Could you check a few things on this drawing? It's one solid part, dimensions in mm from its lowest x, y, z. A direction names the side the tool comes from. Give positions to 0.01 mm unless a question says otherwise; leave off trailing zeros. Order: outer loops, then holes, each group sorted by start corner. A loop starts at its lowest first (then second) coordinate and runs counter-clockwise, first axis right, second up. Notation, with made-up numbers: M 22.5,-15.75 L 38.5,-15.75 A22 ccw 38.5,-5.75 Z; hole C 28.25,88 d6. An arc over 180 degrees is marked long. Use one line per item in the form item = value.
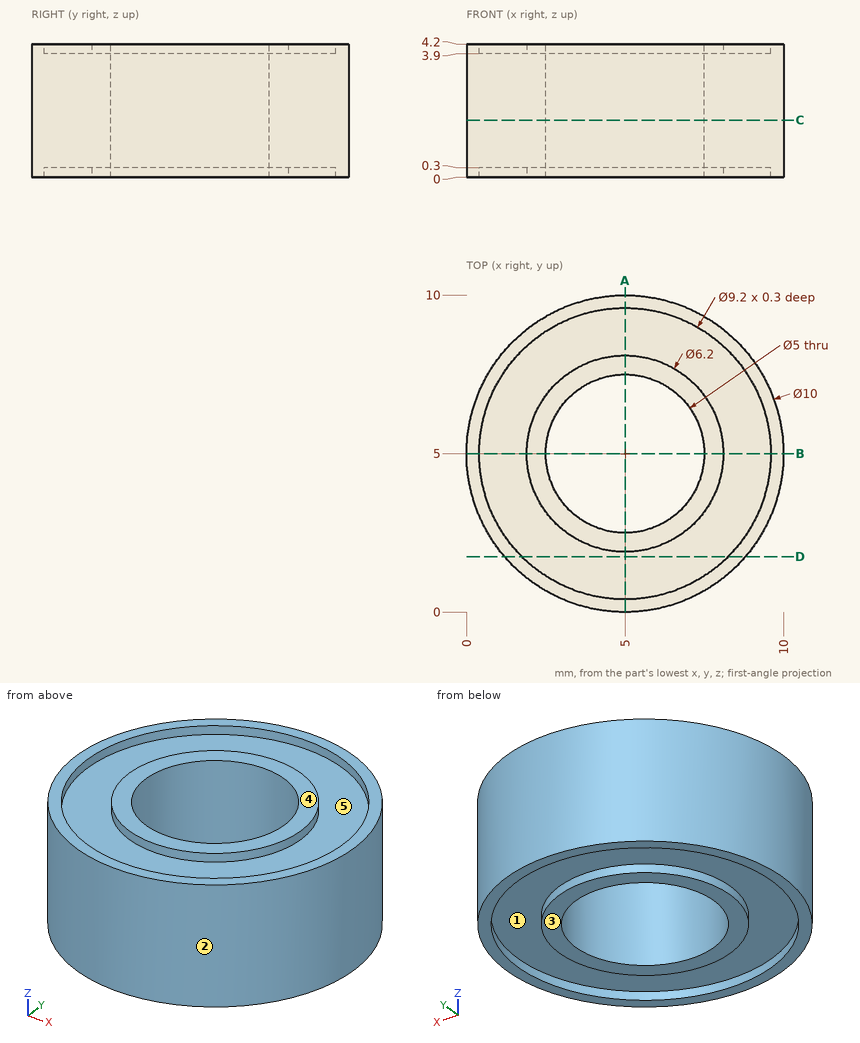
Q1. I want a section at C-C on z = 1.8. Write out the boundary of the cut face in (x, y), then the cut area to 3 significant figures.
Found:
outline = C 5,5 d10; hole C 5,5 d5
area = 58.9 mm²
Q2. I want a section at A-A on x = 5. Write out the boundary of the cut face in (y, z).
Found:
outline = M 0,0 L 0.4,0 L 0.4,0.3 L 1.9,0.3 L 1.9,0 L 2.5,0 L 2.5,4.2 L 1.9,4.2 L 1.9,3.9 L 0.4,3.9 L 0.4,4.2 L 0,4.2 Z; M 7.5,0 L 8.1,0 L 8.1,0.3 L 9.6,0.3 L 9.6,0 L 10,0 L 10,4.2 L 9.6,4.2 L 9.6,3.9 L 8.1,3.9 L 8.1,4.2 L 7.5,4.2 Z
Q3. I need wall thicknesses on L1, parallel to X at y = 5, z = 4.05; L2, parallel to Y at x = 7.75, z = 3.95; L3, parallel to Z at x = 6.75, y = 8.5. Which ranges of each line are inside material? Lowest first, please.
Found:
L1 = 0 to 0.4, 1.9 to 2.5, 7.5 to 8.1, 9.6 to 10
L2 = 0.82 to 1.31, 3.57 to 6.43, 8.69 to 9.18
L3 = 0.3 to 3.9
Q4. I'm going to push a flat-ended pin straight in: pin 1 Ø1 at (x, z) = (7.5, 1) entering from -Y. Where does the tip first touch, or does it pass through?
Found:
pin_1 = 0.42
Q5. I want a section at D-D on y = 1.75. Write out the boundary of the cut face in (x, z).
Found:
outline = M 1.2,0 L 1.74,0 L 1.74,0.3 L 8.26,0.3 L 8.26,0 L 8.8,0 L 8.8,4.2 L 8.26,4.2 L 8.26,3.9 L 1.74,3.9 L 1.74,4.2 L 1.2,4.2 Z
Q6. On a 3-axis mill with a long thin cutter (end or side, diameter ignored), from which of +Z, -Z, +X, -X, +Y, -Y can I reach the whole of each face in a straight line? I mean the marked faces 4 and 5. Say none if no direction works.
Found:
face_4 = +Z, +X, -X, +Y, -Y
face_5 = +Z
Q7. Thinking about a two-plate mould opening in Y: for the marked faces 1, 2 and 3, which applies, +Y half, -Y half, draft (parallel to the pull), parting line (faces both ways), or undercut?
Found:
face_1 = undercut
face_2 = parting line
face_3 = draft
